from build123d import *

# Parameters (mm, degrees)
F0_R     = 5.1
F1_DEPTH = 4


with BuildPart() as f1:
    # F0 (on Front) → F1 (new body)
    with BuildSketch(Plane.XZ):
        with BuildLine():
            ThreePointArc((40, 37.5), (37.803301, 42.803301), (32.5, 45))
            Line((32.5, 45), (-32.5, 45))
            ThreePointArc((-32.5, 45), (-37.803301, 42.803301), (-40, 37.5))
            Line((-40, 37.5), (-40, -45))
            Line((-40, -45), (40, -45))
            Line((40, -45), (40, 37.5))
        make_face()
        with Locations((-25, 30)):
            Circle(F0_R, mode=Mode.SUBTRACT)
        with Locations((0, 5)):
            Circle(F0_R, mode=Mode.SUBTRACT)
        with Locations((25, 30)):
            Circle(F0_R, mode=Mode.SUBTRACT)
    extrude(amount=F1_DEPTH)


solid = f1.part
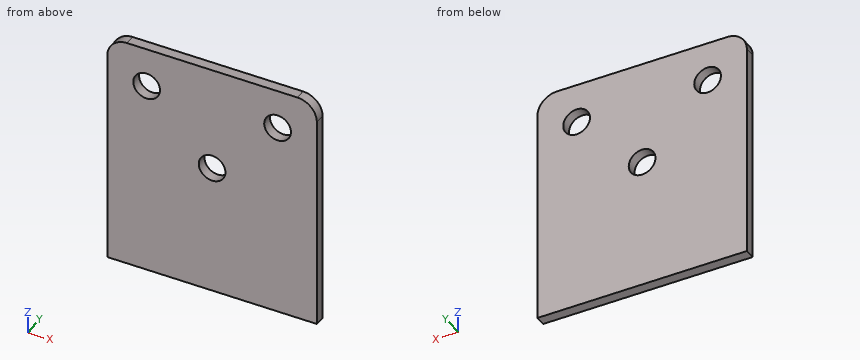
The listing builds one solid part. Answer for the finished solid, in the listing's coordinates (mm). Round coordinates to 2 decimals unless told otherwise and drop trailing zeros. Write each loop counter-clockwise with the first axis right and the second up, starting at its lowest first coordinate (ties: lowest second). Pieces come first, ordered by that corner, then holes. Notation, with made-up numbers: (-8.5, -22) - (35.5, -22) arc R11 ccw to (35.5, -2) - close; hole circle Ø2 at (32, -8.75). An arc over 180 degrees is marked (long way). Use a Markdown table: item, result. Add a question column.
1. A flat-ended cylindrical pin translates along its axis: P1, Ø8, axis at x = 0, z = 5, coming from the +Y side. Find the tip coordinate at first contact, or state that the pin passes through.
2. The part is cut by section B-B (z = 30). Write down the section's boundary in (x, y).
3. The part is cut by section D-D (y = -2.65). Write down the section's boundary in (x, z), and give its area (3 significant figures).
4. The part is cut by section A-A (x = -25). Write down the section's boundary in (y, z).
5. Consider line 1 (Z direction, x = 0, y = -2.3); line 2 (Z direction, x = -25, y = -2.7); line 3 (X direction, y = -1.7, z = 26). Determine where each line is inside the solid, lowest interval first.
6. The part is cut by section C-C (z = 5). Write down the section's boundary in (x, y), and give its area (3 significant figures).
Reported:
| question | item | result |
|---|---|---|
| 1 | P1 | through |
| 2 | outline | (-40, -4) - (-30.1, -4) - (-30.1, 0) - (-40, 0) - close; (-19.9, -4) - (19.9, -4) - (19.9, 0) - (-19.9, 0) - close; (30.1, -4) - (40, -4) - (40, 0) - (30.1, 0) - close |
| 3 | outline | (-40, -45) - (40, -45) - (40, 37.5) arc R7.5 ccw to (32.5, 45) - (-32.5, 45) arc R7.5 ccw to (-40, 37.5) - close; hole circle Ø10.2 at (-25, 30); hole circle Ø10.2 at (0, 5); hole circle Ø10.2 at (25, 30) |
| 3 | area | 6,930 mm^2 |
| 4 | outline | (-4, -45) - (0, -45) - (0, 24.9) - (-4, 24.9) - close; (-4, 35.1) - (0, 35.1) - (0, 45) - (-4, 45) - close |
| 5 | line 1 | -45 to -0.1, 10.1 to 45 |
| 5 | line 2 | -45 to 24.9, 35.1 to 45 |
| 5 | line 3 | -40 to -28.16, -21.84 to 21.84, 28.16 to 40 |
| 6 | outline | (-40, -4) - (-5.1, -4) - (-5.1, 0) - (-40, 0) - close; (5.1, -4) - (40, -4) - (40, 0) - (5.1, 0) - close |
| 6 | area | 279 mm^2 |
